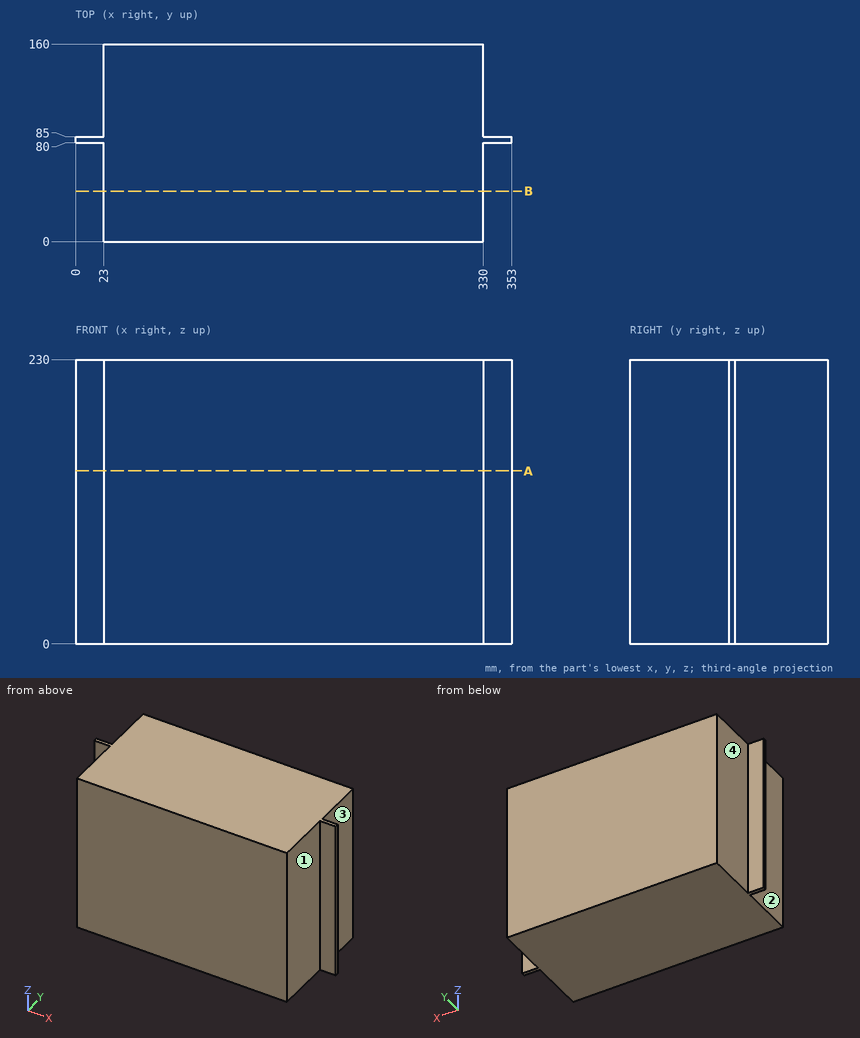
Job drawing, mm, ordinate dimensions from the low corner. One solid piece. A direction names the side the tool comes from. Round coordinates to 2 decimals unless told otherwise and drop trailing zeros. Loops run counter-clockwise (first coordinate to the right, second up) from the corner with the lowest first, then second, coordinate; pieces in that order, holes last.
Item 1: Drop flat-ended pins along their axis: P1, Ø18.5, axis at x = 6.5, z = 137.5, coming from the +Y side; P2, Ø5, axis at y = 102.5, z = 42.5, coming from the -X side; P3, Ø1, axis at y = 90, z = 89, coming from the +X side. Give the stop position or say it passes through.
Item 2: Cut at A-A, the plane z = 140. Give the cut face in (x, y).
Item 3: Cut at B-B, the plane y = 41. Give the cut face in (x, z).
Item 4: 3-axis set-ups, long thin cutter, end or side, ignore diameter. For the marked faces 1, 2, 3 and 4: which of +Z, -Z, +X, -X, +Y, -Y reach the whole face in a straight line?
Item 5: Drill centre line: line 1 (X direction, y = 120, z = 188). Where is it in solid material? Low to high.
A:
1. P1: stops at y = 85
1. P2: stops at x = 23
1. P3: stops at x = 330
2. outline: (0, 80) - (23, 80) - (23, 0) - (330, 0) - (330, 80) - (353, 80) - (353, 85) - (330, 85) - (330, 160) - (23, 160) - (23, 85) - (0, 85) - close
3. outline: (23, 0) - (330, 0) - (330, 230) - (23, 230) - close
4. face 1: +Z, -Z, +X, -Y
4. face 2: +Z, -Z, -X, -Y
4. face 3: +Z, -Z, +X, +Y
4. face 4: +Z, -Z, -X, +Y
5. line 1: x = 23 to 330
